Design review of the part built by this model. Coordinates are the model's own, in mm. Give positions to 0.01 mm unless a question says otherwise; leave off trailing zeros. Write each loop counter-clockwise with the first axis right and the second up, starting at its lowest first coordinate (ties: lowest second). Pieces come first, ordered by that corner, then holes. Notation, with made-up numbers: M 58,16 L 71,16 A21 cw 71,46 Z; hole C -22.5,63.5 d9. An arc over 180 degrees is marked long. Use a Markdown table: item, result. Add a question column.
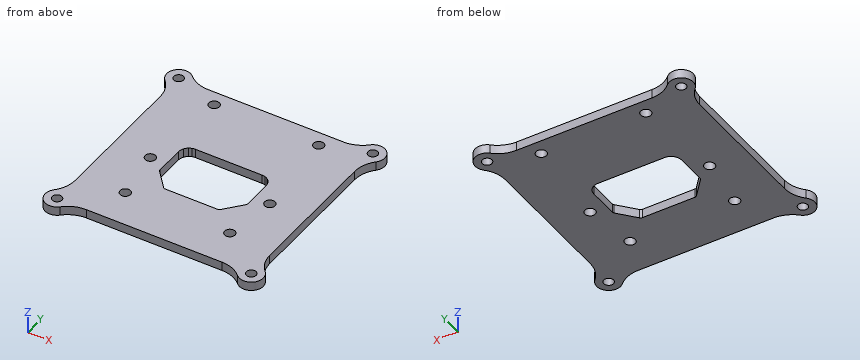
```python
from build123d import *

# Parameters (mm, degrees)
SKETCH_1_R          = 1.625
EXTRUDE_1_DEPTH     = 3
FILLET_1_R          = 10
SKETCH_3_R          = 1.75
CUT_EXTRUDE_1_DEPTH = 10
SKETCH_4_R          = 1.75
CUT_EXTRUDE_2_DEPTH = 10
SKETCH_5_R          = 1.75
CUT_EXTRUDE_3_DEPTH = 10
CUT_EXTRUDE_5_DEPTH = 10


with BuildPart() as part:
    # Эскиз1 → Бобышка-Вытянуть1 (new body)
    with BuildSketch(Plane.XY):
        with BuildLine():
            ThreePointArc((-32.5, -28.5), (-35.328427125, -35.328427125), (-28.5, -32.5))
            Line((-28.5, -32.5), (28.5, -32.5))
            ThreePointArc((28.5, -32.5), (35.328427125, -35.328427125), (32.5, -28.5))
            Line((32.5, -28.5), (32.5, 28.5))
            ThreePointArc((32.5, 28.5), (35.328427125, 35.328427125), (28.5, 32.5))
            Line((28.5, 32.5), (-28.5, 32.5))
            ThreePointArc((-28.5, 32.5), (-35.328427125, 35.328427125), (-32.5, 28.5))
            Line((-32.5, 28.5), (-32.5, -28.5))
        make_face()
        with Locations((-32.5, -32.5)):
            Circle(SKETCH_1_R, mode=Mode.SUBTRACT)
        with Locations((32.5, 32.5)):
            Circle(SKETCH_1_R, mode=Mode.SUBTRACT)
        with Locations((-32.5, 32.5)):
            Circle(SKETCH_1_R, mode=Mode.SUBTRACT)
        with Locations((32.5, -32.5)):
            Circle(SKETCH_1_R, mode=Mode.SUBTRACT)
    extrude(amount=EXTRUDE_1_DEPTH)

    # Скругление1
    fillet_1_edges = [part.edges().sort_by_distance(p)[0] for p in [
        (-32.5, -28.5, 1.5),
        (-32.5, 28.5, 1.5),
        (-28.5, 32.5, 1.5),
        (28.5, 32.5, 1.5),
        (32.5, 28.5, 1.5),
        (32.5, -28.5, 1.5),
        (28.5, -32.5, 1.5),
        (-28.5, -32.5, 1.5),
    ]]
    fillet(fillet_1_edges, radius=FILLET_1_R)

    # Эскиз3 → Вырез-Вытянуть1 (cut)
    with BuildSketch(Plane(origin=(0, 0, 0), x_dir=(-1, 0, 0), z_dir=(0, 0, -1))):
        with Locations((-17.5, 27.5)):
            Circle(SKETCH_3_R)
        with Locations(Location((17.5, 27.5, 0), (0, 0, 180))):
            Circle(SKETCH_3_R)
    extrude(amount=-CUT_EXTRUDE_1_DEPTH, mode=Mode.SUBTRACT)

    # Эскиз4 → Вырез-Вытянуть2 (cut)
    with BuildSketch(Plane(origin=(0, 0, 0), x_dir=(-1, 0, 0), z_dir=(0, 0, -1))):
        with Locations((-20, -2.615263412)):
            Circle(SKETCH_4_R)
        with Locations(Location((20, -2.615263412, 0), (0, 0, 180))):
            Circle(SKETCH_4_R)
    extrude(amount=-CUT_EXTRUDE_2_DEPTH, mode=Mode.SUBTRACT)

    # Эскиз5 → Вырез-Вытянуть3 (cut)
    with BuildSketch(Plane.XY.offset(3)):
        with Locations((-17.5, -20)):
            Circle(SKETCH_5_R)
        with Locations((17.5, -20)):
            Circle(SKETCH_5_R)
    extrude(amount=-CUT_EXTRUDE_3_DEPTH, mode=Mode.SUBTRACT)

    # Эскиз6 → Вырез-Вытянуть5 (cut)
    with BuildSketch(Plane.XY.offset(3)):
        with BuildLine():
            ThreePointArc((-14.17, 3.884736588), (-13.825652378, 5.280268906), (-12.871659701, 6.355435733))
            Line((-12.871659701, 6.355435733), (-14.131289938, 5.750416599))
            ThreePointArc((-14.131289938, 5.750416599), (-14.532626561, 4.855685922), (-14.67, 3.884736588))
            Line((-14.67, 3.884736588), (-14.67, -5.929561494))
            ThreePointArc((-14.67, -5.929561494), (-14.607432841, -6.277727646), (-14.427560661, -6.582326264))
            Line((-14.427560661, -6.582326264), (-9.528380842, -12.268028181))
            ThreePointArc((-9.528380842, -12.268028181), (-9.187494653, -12.524319177), (-8.770820181, -12.615263412))
            Line((-8.770820181, -12.615263412), (8.770820181, -12.615263412))
            ThreePointArc((8.770820181, -12.615263412), (9.187494653, -12.524319177), (9.528380842, -12.268028181))
            Line((9.528380842, -12.268028181), (14.427560661, -6.582326264))
            ThreePointArc((14.427560661, -6.582326264), (14.607432841, -6.277727646), (14.67, -5.929561494))
            Line((14.67, -5.929561494), (14.67, 3.884736588))
            ThreePointArc((14.67, 3.884736588), (14.532626561, 4.855685922), (14.131289938, 5.750416599))
            Line((14.131289938, 5.750416599), (12.871659701, 6.355435733))
            ThreePointArc((12.871659701, 6.355435733), (13.825652378, 5.280268906), (14.17, 3.884736588))
            Line((14.17, 3.884736588), (14.17, -5.929561494))
            ThreePointArc((14.17, -5.929561494), (14.13871642, -6.10364457), (14.048780331, -6.255943879))
            Line((14.048780331, -6.255943879), (9.149600512, -11.941645796))
            ThreePointArc((9.149600512, -11.941645796), (8.979157417, -12.069791294), (8.770820181, -12.115263412))
            Line((8.770820181, -12.115263412), (-8.770820181, -12.115263412))
            ThreePointArc((-8.770820181, -12.115263412), (-8.979157417, -12.069791294), (-9.149600512, -11.941645796))
            Line((-9.149600512, -11.941645796), (-14.048780331, -6.255943879))
            ThreePointArc((-14.048780331, -6.255943879), (-14.13871642, -6.10364457), (-14.17, -5.929561494))
            Line((-14.17, -5.929561494), (-14.17, 3.884736588))
        make_face()
        with BuildLine():
            Line((11.17, 7.384736588), (10.728688662, 7.384736588))
            Line((10.728688662, 7.384736588), (12.034826728, 6.757379053))
            ThreePointArc((12.034826728, 6.757379053), (12.468885198, 6.588973494), (12.871659701, 6.355435733))
            Line((12.871659701, 6.355435733), (14.131289938, 5.750416599))
            ThreePointArc((14.131289938, 5.750416599), (13.694992017, 6.308455903), (13.155269651, 6.767218923))
            add(Edge.make_bspline(
                [(12.178964517, 7.236152797), (12.708169697, 7.084996084), (13.155269651, 6.767218923)],
                knots=[0, 0, 0, 1, 1, 1], degree=2))
            ThreePointArc((12.178964517, 7.236152797), (11.679923165, 7.347391403), (11.17, 7.384736588))
        make_face()
        with BuildLine():
            Line((-10.728688662, 7.384736588), (-12.034826728, 6.757379053))
            ThreePointArc((-12.034826728, 6.757379053), (-11.607076999, 6.85272643), (-11.17, 6.884736588))
            Line((-11.17, 6.884736588), (11.17, 6.884736588))
            ThreePointArc((11.17, 6.884736588), (11.607076999, 6.85272643), (12.034826728, 6.757379053))
            Line((12.034826728, 6.757379053), (10.728688662, 7.384736588))
            Line((10.728688662, 7.384736588), (-10.728688662, 7.384736588))
        make_face()
        with BuildLine():
            Line((-14.131289938, 5.750416599), (-12.871659701, 6.355435733))
            ThreePointArc((-12.871659701, 6.355435733), (-12.468885198, 6.588973494), (-12.034826728, 6.757379053))
            Line((-12.034826728, 6.757379053), (-10.728688662, 7.384736588))
            Line((-10.728688662, 7.384736588), (-11.17, 7.384736588))
            ThreePointArc((-11.17, 7.384736588), (-11.679923165, 7.347391403), (-12.178964517, 7.236152797))
            add(Edge.make_bspline(
                [(-12.178964517, 7.236152797), (-12.706483, 7.080112966), (-13.155269651, 6.767218923)],
                knots=[0, 0, 0, 1, 1, 1], degree=2))
            ThreePointArc((-13.155269651, 6.767218923), (-13.694992017, 6.308455903), (-14.131289938, 5.750416599))
        make_face()
    extrude(amount=-CUT_EXTRUDE_5_DEPTH, mode=Mode.SUBTRACT)


with BuildPart() as body_2:
    # of the pieces the cut leaves, the one that is kept (cut_extrude_5_keep)
    add(part.part.solids().sort_by_distance((-32.5, 22.702041029, 0))[0])


solid = body_2.part
```
(1) Wall thickness on L1, parallel to Y at x = 17.5, z = 2.35; L2, parallel to X at y = -2, z = 0.6; L3, parallel to X at y = -0.5, z = 0.55: over which ranges is each line inside the solid? List them lowest first.
(2) Add section C-C on x = 3. Give the boundary of the cut face in (y, z).
(3) Add section A-A on y = -20. Give the boundary of the cut face in (x, z).
(4) Add section B-B on y = 1. Give the boundary of the cut face in (x, z), then the cut area to 3 significant figures.
(5) Add section D-D on z = 1.2. Give the number of separate pieces and of enclosed holes in the cut face, then the cut area to 3 significant figures.
(6) For pin 1 (1.5 mm diameter, centred on x = -22, z = 2.5, fed in from +Y); pin 2 (0.9 mm diameter, centred on y = -5.5, z = 1.5, fed in from +X); pin 3 (1.5 mm diameter, centred on x = -1, z = 1.5, fed in from -Y), all flat-tipped, find the tip position at first contact; note any pin that passes through.
From the geometry:
| question | item | result |
|---|---|---|
| 1 | L1 | y = -32.5 to -21.75, -18.25 to 25.75, 29.25 to 32.5 |
| 1 | L2 | x = -32.5 to -21.64, -18.36 to -14.67, 14.67 to 18.36, 21.64 to 32.5 |
| 1 | L3 | x = -32.5 to -14.67, 14.67 to 32.5 |
| 2 | outline | M -32.5,0 L -12.62,0 L -12.62,3 L -32.5,3 Z; M 7.38,0 L 32.5,0 L 32.5,3 L 7.38,3 Z |
| 3 | outline | M -32.5,0 L -19.25,0 L -19.25,3 L -32.5,3 Z; M -15.75,0 L 15.75,0 L 15.75,3 L -15.75,3 Z; M 19.25,0 L 32.5,0 L 32.5,3 L 19.25,3 Z |
| 4 | outline | M -32.5,0 L -14.67,0 L -14.67,3 L -32.5,3 Z; M 14.67,0 L 32.5,0 L 32.5,3 L 14.67,3 Z |
| 4 | area | 107 mm^2 |
| 5 | separate pieces | 1 |
| 5 | enclosed holes | 11 |
| 5 | area | 3,770 mm^2 |
| 6 | pin 1 | stops at y = 32.5 |
| 6 | pin 2 | stops at x = 32.5 |
| 6 | pin 3 | stops at y = -32.5 |
